from build123d import *

# Parameters (mm, degrees)
EXTRUDE_DEPTH               = 5
EXTRUDE001_DEPTH            = 5
THICKNESS_T                 = 1
BOX004_W                    = 5
BOX004_H                    = 5
BOX004_DEPTH                = 5
CYLINDER001_W               = 48
CYLINDER001_H               = 15
CYLINDER001_ANGLE           = 60
CYLINDER001_PLACEMENT_ANGLE = 60
CYLINDER_W                  = 51
CYLINDER_H                  = 15
CYLINDER_ANGLE              = 60
CYLINDER_PLACEMENT_ANGLE    = 60
BOX003_W                    = 6
BOX003_H                    = 4
BOX003_DEPTH                = 15
BOX002_W                    = 12
BOX002_H                    = 10
BOX002_DEPTH                = 15
BOX001_W                    = 13
BOX001_H                    = 22
BOX001_DEPTH                = 12
BOX_W                       = 15
BOX_H                       = 34
BOX_DEPTH                   = 14


with BuildPart() as extrude_body:
    with BuildSketch(Plane(origin=(8.5, 45, 6), x_dir=(1, 0, 0), z_dir=(0, 1, 0))):
        with BuildLine():
            Line((5, 4), (-5, 4))
            Line((-5, 4), (-5, -3.142136))
            ThreePointArc((-5, -3.142136), (-2.53653, -3.783978), (0, -4))
            ThreePointArc((0, -4), (2.53653, -3.783978), (5, -3.142136))
            Line((5, -3.142136), (5, 4))
        make_face()
    extrude(amount=EXTRUDE_DEPTH)


with BuildPart() as extrude001:
    with BuildSketch(Plane(origin=(8.5, 45, 6), x_dir=(1, 0, 0), z_dir=(0, 1, 0))):
        with BuildLine():
            Line((5, 4), (-5, 4))
            Line((-5, 4), (-5, -3.142136))
            ThreePointArc((-5, -3.142136), (-2.53653, -3.783978), (0, -4))
            ThreePointArc((0, -4), (2.53653, -3.783978), (5, -3.142136))
            Line((5, -3.142136), (5, 4))
        make_face()
    extrude(amount=EXTRUDE001_DEPTH)


with BuildPart() as fusion001:
    # Thickness base: copy of Extrude body
    add(extrude_body.part)

    # Thickness
    thickness_openings = [fusion001.faces().sort_by_distance(p)[0] for p in [
        (8.5, 50, 5.862901),
    ]]
    offset(amount=THICKNESS_T, openings=thickness_openings)

    # Fusion001: union Extrude body, Extrude001
    add(extrude_body.part)
    add(extrude001.part)


with BuildPart() as fusion001_1:
    # Fusion001 placement: moved
    add(fusion001.part.moved(Location((0, -7, 1))))


with BuildPart() as pin_opening:
    # Box004 → Box004 (new body)
    with BuildSketch(Plane(origin=(6, 38.5, 5), x_dir=(1, 0, 0), z_dir=(0, 0, 1))):
        with Locations((2.5, 2.5)):
            Rectangle(BOX004_W, BOX004_H)
    extrude(amount=BOX004_DEPTH)


with BuildPart() as bottle_wall001:
    # Cylinder001 → Cylinder001 (revolve)
    with BuildSketch(Plane.XZ):
        with Locations((24, 7.5)):
            Rectangle(CYLINDER001_W, CYLINDER001_H)
    revolve(axis=Axis((0, 0, 0), (0, 0, 1)), revolution_arc=CYLINDER001_ANGLE)


with BuildPart() as bottle_wall001_1:
    # Cylinder001 placement: moved
    add(bottle_wall001.part.moved(Location((8.5, -7, 0))).rotate(Axis((8.5, -7, 0), (0, 0, 1)), CYLINDER001_PLACEMENT_ANGLE))


with BuildPart() as cut005:
    # Cylinder → Cylinder (revolve)
    with BuildSketch(Plane.XZ):
        with Locations((25.5, 7.5)):
            Rectangle(CYLINDER_W, CYLINDER_H)
    revolve(axis=Axis((0, 0, 0), (0, 0, 1)), revolution_arc=CYLINDER_ANGLE)


with BuildPart() as cut005_1:
    # Cylinder placement: moved
    add(cut005.part.moved(Location((8.5, -7, 0))).rotate(Axis((8.5, -7, 0), (0, 0, 1)), CYLINDER_PLACEMENT_ANGLE))

    # Cut005: cut bottle_wall001
    add(bottle_wall001_1.part, mode=Mode.SUBTRACT)


with BuildPart() as cut005_2:
    # Cut005 placement: moved
    add(cut005_1.part.moved(Location((0, -2, 0))))


with BuildPart() as cone:
    # Cone → Cone (revolve)
    with BuildSketch(Plane(origin=(8.5, 7, 2), x_dir=(1, 0, 0), z_dir=(0, -1, 0))):
        Polygon((0, 0), (1, 0), (2, 5), (0, 5), align=None)
    revolve(axis=Axis((8.5, 7, 2), (0, 0, 1)))


with BuildPart() as pinhole:
    # Sphere → Sphere (revolve)
    with BuildSketch(Plane(origin=(8.5, 7.25, 7), x_dir=(1, 0, 0), z_dir=(0, -1, 0))):
        with BuildLine():
            ThreePointArc((0, -3.5), (3.5, 0), (0, 3.5))
            Line((0, 3.5), (0, -3.5))
        make_face()
    revolve(axis=Axis((8.5, 7.25, 7), (0, 0, 1)))


with BuildPart() as neck:
    # Box003 → Box003 (new body)
    with BuildSketch(Plane(origin=(5.5, 28, 4), x_dir=(1, 0, 0), z_dir=(0, 0, 1))):
        with Locations((3, 2)):
            Rectangle(BOX003_W, BOX003_H)
    extrude(amount=BOX003_DEPTH)


with BuildPart() as pullbay:
    # Box002 → Box002 (new body)
    with BuildSketch(Plane(origin=(2.5, 30, 2), x_dir=(1, 0, 0), z_dir=(0, 0, 1))):
        with Locations((6, 5)):
            Rectangle(BOX002_W, BOX002_H)
    extrude(amount=BOX002_DEPTH)


with BuildPart() as solenoidbay:
    # Box001 → Box001 (new body)
    with BuildSketch(Plane(origin=(2, 7, 2), x_dir=(1, 0, 0), z_dir=(0, 0, 1))):
        with Locations((6.5, 11)):
            Rectangle(BOX001_W, BOX001_H)
    extrude(amount=BOX001_DEPTH)


with BuildPart() as cut007:
    # Box → Box (new body)
    with BuildSketch(Plane(origin=(1, 6, 0), x_dir=(1, 0, 0), z_dir=(0, 0, 1))):
        with Locations((7.5, 17)):
            Rectangle(BOX_W, BOX_H)
    extrude(amount=BOX_DEPTH)

    # Cut: cut solenoidBay
    add(solenoidbay.part, mode=Mode.SUBTRACT)

    # Cut001: cut pullBay
    add(pullbay.part, mode=Mode.SUBTRACT)

    # Cut002: cut neck
    add(neck.part, mode=Mode.SUBTRACT)

    # Cut003: cut pinhole
    add(pinhole.part, mode=Mode.SUBTRACT)

    # Cut004: cut Cone
    add(cone.part, mode=Mode.SUBTRACT)

    # Fusion: union Cut005
    add(cut005_2.part)

    # Cut006: cut pin_opening
    add(pin_opening.part, mode=Mode.SUBTRACT)

    # Cut007: cut Fusion001
    add(fusion001_1.part, mode=Mode.SUBTRACT)


solid = cut007.part
The listing builds one solid part. Answer for the finished solid, in the listing's coordinates (mm). A direction names the side the tool comes from. Round coordinates to 2 decimals unless told otherwise and drop trailing zeros. Order: outer loops, then holes, each group sorted by start corner. A loop starts at its lowest first (then second) coordinate and runs counter-clockwise, first axis right, second up. Notation, with made-up numbers: (48.25, 75.25) -> (84.25, 75.25) arc R14 cw to (84.25, 101.25) -> close; hole circle Ø2 at (56, 49). An arc over 180 degrees is marked (long way). Put each result on its own line as item: value.
Q1. Section A-A, the plane z = 13.25 is taken. Write down the section's boundary in (x, y), and give its area (3 significant figures).
Results list:
outline: (-17, 35.17) -> (-15.5, 32.57) arc R48 cw to (1, 38.41) -> (1, 6) -> (16, 6) -> (16, 38.41) arc R48 cw to (32.5, 32.57) -> (34, 35.17) arc R51 ccw to start; hole (2, 7) -> (15, 7) -> (15, 29) -> (11.5, 29) -> (11.5, 30) -> (14.5, 30) -> (14.5, 38.62) arc R48 ccw to (2.5, 38.62) -> (2.5, 30) -> (5.5, 30) -> (5.5, 29) -> (2, 29) -> close
area: 249 mm^2
Q2. Section D-D, the plane y = 13 is taken. Write down the section's boundary in (x, z), and give its area (3 significant figures).
Results list:
outline: (1, 0) -> (16, 0) -> (16, 14) -> (15, 14) -> (15, 2) -> (2, 2) -> (2, 14) -> (1, 14) -> close
area: 54.0 mm^2
Q3. Section B-B, the plane y = 37 is taken. Write down the section's boundary in (x, z).
Results list:
outline: (-13.52, 0) -> (-5.21, 0) -> (-5.21, 15) -> (-13.52, 15) -> close; (1, 0) -> (16, 0) -> (16, 14) -> (14.5, 14) -> (14.5, 2) -> (2.5, 2) -> (2.5, 14) -> (1, 14) -> close; (22.21, 0) -> (30.52, 0) -> (30.52, 15) -> (22.21, 15) -> close
Q4. Consider line 1 along Y through (x, z) = (12, 12); line 2 along X through (y, z) = (24.5, 11); line 3 along Y through (x, z) = (5, 2.5). Determine where each line is inside the solid, lowest interval first.
Results list:
line 1: 6 to 7, 29 to 30, 38.87 to 41.88
line 2: 1 to 2, 15 to 16
line 3: 6 to 7, 29 to 30
Q5. Section C-C, the plane z = 8.5 is taken. Write down the section's boundary in (x, y), and give its area (3 significant figures).
Results list:
outline: (-17, 35.17) -> (-15.5, 32.57) arc R48 cw to (1, 38.41) -> (1, 6) -> (5.6, 6) arc R3.16 cw to (5.35, 7) -> (2, 7) -> (2, 29) -> (5.5, 29) -> (5.5, 30) -> (2.5, 30) -> (2.5, 41.65) arc R51 ccw to start; (11.4, 6) -> (16, 6) -> (16, 38.41) arc R48 cw to (32.5, 32.57) -> (34, 35.17) arc R51 ccw to (14.5, 41.65) -> (14.5, 30) -> (11.5, 30) -> (11.5, 29) -> (15, 29) -> (15, 7) -> (11.65, 7) arc R3.16 cw to start
area: 207 mm^2
Q6. Which of the six approach directions +Z, -Z, +X, -X, +Y, -Y give full straight-line access (tool end or side, diameter ignored) to faces 1 (the flat face through (9, 36, 2)), 2 (the flat face through (8.5, 29.5, 4)), 3 (the flat face through (8, 7, 11)), 4 (the cylindrical face through (2.801, 40.211, 2.285))?
Results list:
face 1: none
face 2: +Z, +Y
face 3: +Z
face 4: +Y
Q7. Determine the mould class of faces 5 (the flat face through (33.24, 33.85, 7.6)), 6 (the flat face through (15, 18, 8)), 7 (the flat face through (-16.24, 33.85, 7.6)), 8 (the conical face through (7.518, 6.328, 2.948)) for opening direction X: pulls with the +X half, pulls with the -X half, needs draft (parallel to the pull), parting line crosses it, or undercut.
Results list:
face 5: pulls with the +X half
face 6: undercut
face 7: pulls with the -X half
face 8: undercut
Q8. Each of these flat-tipped pins is pushed along its axis until it touches: P1, Ø1.5, axis at x = -7, z = 3, coming from the -Y side; P2, Ø3.5, axis at y = 16.5, z = 9.5, coming from the -X side; P3, Ø3.5, axis at x = 9.5, z = 9.5, coming from the +Y side. Where does it stop, or does it pass through?
Results list:
P1: y = 36.17
P2: x = 1
P3: y = 7
